Geometry check sheet. Reference: the model listing, model coordinates, mm. A direction names the side the tool comes from. Round coordinates to 2 decimals unless told otherwise and drop trailing zeros. Write each loop counter-clockwise with the first axis right and the second up, starting at its lowest first coordinate (ties: lowest second). Pieces come first, ordered by that corner, then holes. Notation, with made-up numbers: M 23.5,51 L 33.5,51 A17 cw 33.5,77 Z; hole C 22.25,-3 d4. An arc over 180 degrees is marked long. Use a Markdown table: item, result.
Autodesk Inventor part; units mm, degrees
ref_plane "YZ Plane" through (0, 0, 0) normal (1, 0, 0) x (0, 1, 0)
ref_plane "XZ Plane" through (0, 0, 0) normal (0, 1, 0) x (-1, 0, 0)
ref_plane "XY Plane" through (0, 0, 0) normal (0, 0, 1) x (1, 0, 0)
sketch "Sketch1" plane through (0, 0, 0) normal (0, 0, 1) x (1, 0, 0)
  line L0 (-29.5214, 15.9367) -> (33.9786, 15.9367)
  line L1 (33.9786, 15.9367) -> (33.9786, -28.5133)
  line L2 (33.9786, -28.5133) -> (-29.5214, -28.5133)
  line L3 (-29.5214, -28.5133) -> (-29.5214, 15.9367)
  point P0 (0, 0)
  dimension "d0" = 63.5
  dimension "d1" = 44.45
extrude "Extrusion1" add sketch "Sketch1" along normal blind 25.4
sketch "Sketch2" plane through (0, 0, 25.4) normal (0, 0, 1) x (1, 0, 0)
  line L0 (33.9786, 15.9367) -> (-29.5214, 15.9367)
  line L1 (-29.5214, -28.5133) -> (33.9786, -28.5133)
  line L2 (-10.4714, 15.9367) -> (33.9786, 15.9367)
  line L3 (33.9786, 15.9367) -> (33.9786, -28.5133)
  line L4 (-10.4714, 15.9367) -> (21.2786, -28.5133)
  point P0 (0, 0)
  dimension "d4" = 19.05
  dimension "d12" = 12.7
extrude "Extrusion2" cut sketch "Sketch2" against normal blind 12.7
sketch "Sketch3" plane through (0, 0, 25.4) normal (0, 0, 1) x (1, 0, 0)
  line L0 (33.9786, -28.5133) -> (-29.5214, -28.5133)
  line L1 (33.9786, -28.5133) -> (8.5786, -28.5133)
  circle A0 centre (-4.1214, -3.1133) radius 12.7
  line L2 (-29.5214, 15.9367) -> (-29.5214, -28.5133)
  point P0 (0, 0)
  dimension "d14" = 25.4
  dimension "d15" = 25.4
  dimension "d16" = 25.4
extrude "Extrusion3" cut sketch "Sketch3" against normal blind 25.4
Item 1: Material ranges on line 1 along Z through (x, y) = (29.5, 0); line 2 along X through (y, z) = (7, 12); line 3 along X through (y, z) = (-3.5, 10.5), recorded low to high. Write a range as from..to.
Outcome:
| item | result |
|---|---|
| line 1 | z = 0..12.7 |
| line 2 | x = -29.52..-11.8, 3.56..33.98 |
| line 3 | x = -29.52..-16.82, 8.57..33.98 |
Item 2: Cross-section at D-D, the plane x = 29. Record the cut outline in (y, z), and give its area (3 significant figures).
Outcome:
| item | result |
|---|---|
| outline | M -28.51,0 L 15.94,0 L 15.94,12.7 L -28.51,12.7 Z |
| area | 565 mm2 |
Item 3: Cross-section at C-C, the plane z = 2.5. Record the cut outline in (x, y), and give its area (3 significant figures).
Outcome:
| item | result |
|---|---|
| outline | M -29.52,-28.51 L 33.98,-28.51 L 33.98,15.94 L -29.52,15.94 Z; hole C -4.12,-3.11 d25.4 |
| area | 2,320 mm2 |
Item 4: Mould release check, pull along Y, two halves, no side actions. Record for faces 3 (the face through (-14.2, -10.84, 10.06)), 4 (the face through (9, -6, 0)), 5 (the face through (-5, 15.937, 10)): +Y half, -Y half, draft (parallel to the pull), parting line (faces both ways), or undercut.
Outcome:
| item | result |
|---|---|
| face 3 | undercut |
| face 4 | draft |
| face 5 | +Y half |
Item 5: Go/stop test with a flat-tipped pin: pin 1 (3 mm diameter, centred on x = 17.5, y = 2, fed in from -Z). Record where the tip stops, or that it passes through.
Outcome:
| item | result |
|---|---|
| pin 1 | stops at z = 0 |
Item 6: Cross-section at A-A, the plane x = 4. Record the cut outline in (y, z).
Outcome:
| item | result |
|---|---|
| outline | M -28.51,0 L -12.88,0 L -12.88,25.4 L -28.51,25.4 Z; M 6.65,0 L 15.94,0 L 15.94,12.7 L 6.65,12.7 Z |
Item 7: Cross-section at B-B, the plane y = -4. Record the cut outline in (x, z).
Outcome:
| item | result |
|---|---|
| outline | M -29.52,0 L -16.79,0 L -16.79,25.4 L -29.52,25.4 Z; M 8.55,0 L 33.98,0 L 33.98,12.7 L 8.55,12.7 Z |
Item 8: Access from +Z, -Z, +X, -X, +Y, -Y to the whole of each face (thin tool, end or side, straight path). Record for faces 1 (the face through (-29.521, -7, 13)), 2 (the face through (21, -1, 12.7)).
Outcome:
| item | result |
|---|---|
| face 1 | +Z, -Z, -X, +Y, -Y |
| face 2 | +Z, +X, +Y |
